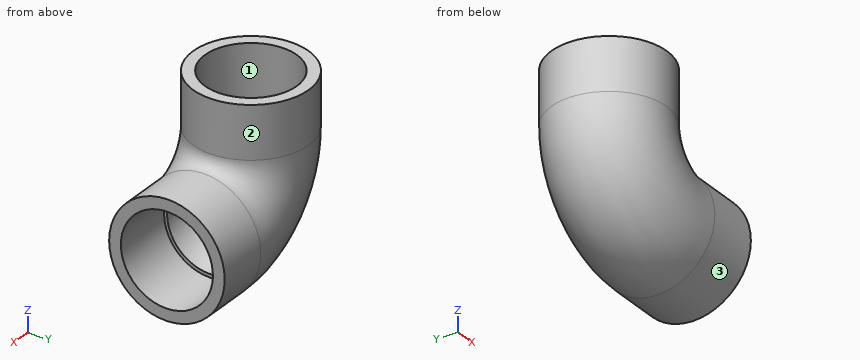
```python
from build123d import *

# Parameters (mm, degrees)
SKETCH1_R          = 20.955
SKETCH1_R_2        = 15.621
SKETCH17_R         = 16.7005
CUT_EXTRUDE1_DEPTH = 22.86
SKETCH18_R         = 16.7005
CUT_EXTRUDE2_DEPTH = 22.86


with BuildPart() as part:
    # Sweep7: sweep along a path in Sketch15
    with BuildLine(Plane(origin=(0, 0, 0), x_dir=(1, 0, 0), z_dir=(0, 1, 0))) as sweep7_path:
        Line((0, 0), (0, 19.05))
        ThreePointArc((0, 19.05), (7.439487758, 37.010512242), (25.4, 44.45))
        Line((25.4, 44.45), (44.45, 44.45))
    # Sketch1 → Sweep7 (sweep)
    with BuildSketch(Plane.XY):
        Circle(SKETCH1_R)
        Circle(SKETCH1_R_2, mode=Mode.SUBTRACT)
    sweep(path=sweep7_path.line)

    # Sketch17 → Cut-Extrude1 (cut)
    with BuildSketch(Plane.XY):
        Circle(SKETCH17_R)
    extrude(amount=-CUT_EXTRUDE1_DEPTH, mode=Mode.SUBTRACT)

    # Sketch18 → Cut-Extrude2 (cut)
    with BuildSketch(Plane(origin=(44.45, 0, 0), x_dir=(0, 0, -1), z_dir=(1, 0, 0))):
        with Locations((44.45, 0)):
            Circle(SKETCH18_R)
    extrude(amount=-CUT_EXTRUDE2_DEPTH, mode=Mode.SUBTRACT)


solid = part.part
```
For this review, take the finished solid that the model builds, in its own axes (mm). Face numbers are marked on the shaded views. Give positions to 0.01 mm unless a question says otherwise; leave off trailing zeros. Write each loop counter-clockwise with the first axis right and the second up, starting at its lowest first coordinate (ties: lowest second). Pieces come first, ordered by that corner, then holes. Notation, with made-up numbers: M 80,13 L 128,13 A17 ccw 128,22 Z; hole C 27.25,19.5 d11. An arc over 180 degrees is marked long. Answer as a JSON object with one key per item and string values. Group by question number.
Item 1: Draft analysis for pull direction X (two halves, no side actions). For the marked faces 1, 2 and 3, state which applies: +X half, -X half, draft (parallel to the pull), parting line (faces both ways), or undercut.
Item 2: Consider section C-C on z = -12. Write out the cut boundary in (x, y) (1 decimal), plus the area to 3 significant figures.
Item 3: Consider section A-A on y = 3. Write out the cut boundary in (x, z).
Item 4: For probe 1 along Y at (x, z) = (0, -15.25) (1 decimal); probe 2 along Y at (x, z) = (27, -44); probe 3 along X at (y, z) = (-6, -9), list the stretches that pass through material, from the lowest coordinate up. Write a range as [from, to].
Item 5: Consider section D-D on y = 9. Write out the cut boundary in (x, z).
Item 6: For pin 1 Ø1 at (x, y) = (-9, 7) entering from +Z; pin 2 Ø6 at (x, z) = (28.5, -44.5) entering from -Y (3 decimals); pin 3 Ø6 at (x, z) = (31, -26.5) entering from -Y, all flat-tipped, find the tip position at first contact; note any pin that passes through.
Check result:
{
 "1": {"face 1": "undercut", "face 2": "parting line", "face 3": "draft"},
 "2": {"outline": "C 0,0 d41.9; hole C 0,0 d33.4", "area": "503 mm^2"},
 "3": {"outline": "M -20.74,-19.05 A46.14 ccw 25.4,-65.19 L 44.45,-65.19 L 44.45,-60.88 L 21.59,-60.88 L 21.59,-59.6 A40.73 cw -15.15,-22.86 L -16.43,-22.86 L -16.43,0 L -20.74,0 Z; M 16.08,-22.86 A10.07 ccw 21.59,-28.37 L 21.59,-28.02 L 44.45,-28.02 L 44.45,-23.71 L 25.4,-23.71 A4.66 cw 20.74,-19.05 L 20.74,0 L 16.43,0 L 16.43,-22.86 Z"},
 "4": {"probe 1": "y = [-21, -16.7], [16.7, 21]", "probe 2": "y = [-20.95, -16.69], [16.69, 20.95]", "probe 3": "x = [-20.08, -15.59], [15.59, 20.08]"},
 "5": {"outline": "M -18.92,-19.05 A44.32 ccw 25.4,-63.37 L 44.45,-63.37 L 44.45,-58.52 L 21.59,-58.52 L 21.59,-57.03 A38.17 cw -12.58,-22.86 L -14.07,-22.86 L -14.07,0 L -18.92,0 Z; M 13.36,-22.86 A12.63 ccw 21.59,-31.09 L 21.59,-30.38 L 44.45,-30.38 L 44.45,-25.53 L 25.4,-25.53 A6.48 cw 18.92,-19.05 L 18.92,0 L 14.07,0 L 14.07,-22.86 Z"},
 "6": {"pin 1": "stops at z = -37.11", "pin 2": "stops at y = -20.955", "pin 3": "stops at y = -14.68"}
}
